Geometry: final body of the model. Coordinates: model frame, mm. Round coordinates to 2 decimals unless told otherwise and drop trailing zeros. Loops run counter-clockwise (first coordinate to the right, second up) from the corner with the lowest first, then second, coordinate; pieces in that order, holes last. Notation, with made-up numbers: (20, 76) - (68, 76) arc R23 ccw to (68, 93) - close; hole circle Ø5 at (-8, 76.5). An arc over 180 degrees is marked (long way). Write item = value, one per line. Start each with the question number.
Item 1: Section A-A (x = 5). Return loops of the section in (y, z).
Item 2: First-contact query: pin 1 (10 mm diameter, centred on y = 30.5, z = 30.5, fed in from +X); pin 2 (3 mm diameter, centred on y = 31.5, z = 99.5, fed in from +X); pin 3 (5 mm diameter, centred on x = 11, z = 122.5, fed in from -Y). Flat tips, straight axial feed; report the tip coordinate or a pass-through.
Item 3: Section C-C (z = 54). Return loops of the section in (x, y).
Item 4: Line query: line 1 (Z direction, x = 3.5, y = 28.5); line 2 (X direction, y = 20.5, z = 25); line 3 (Y direction, x = 1.75, z = 95.5) (3 decimals). Output: solid intervals per line, ascending. Write a range as from..to.
Item 5: Section B-B (y = 34.5). Return loops of the section in (x, z).
from build123d import *

# Parameters (mm, degrees)
F1_DEPTH = 12.7
F2_R     = 3.175
F3_DEPTH = 25.4
F5_DEPTH = 254


with BuildPart() as f1:
    # F0 (on Right) → F1 (new body)
    with BuildSketch(Plane.YZ):
        Polygon((19.05, 127), (0, 0), (38.1, 0), (38.1, 152.4), align=None)
    extrude(amount=F1_DEPTH)

    # F2 (on face) → F3 (cut)
    with BuildSketch(Plane(origin=(0, 0, 0), x_dir=(1, 0, 0), z_dir=(0, 0, -1))):
        with Locations((5.715, -22.225)):
            Circle(F2_R)
    extrude(amount=-F3_DEPTH, mode=Mode.SUBTRACT)

    # F4 (on face) → F5 (cut)
    with BuildSketch(Plane(origin=(0, 0, 0), x_dir=(1, 0, 0), z_dir=(0, 0, -1))):
        Polygon((6.35, 0), (12.7, -38.1), (12.7, 0), align=None)
    extrude(amount=-F5_DEPTH, mode=Mode.SUBTRACT)


solid = f1.part
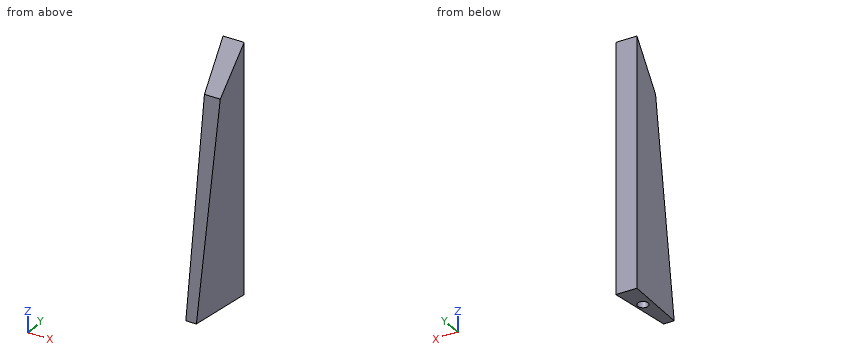
Taken from the geometry:
q1.outline = (0, 0) - (19.13, 0) - (19.13, 25.4) - (25.32, 25.4) - (25.32, 0) - (38.1, 0) - (38.1, 152.4) - (19.05, 127) - close
q2.pin_1 = 12.27
q2.pin_2 = 11.85
q2.pin_3 = 18.09
q3.outline = (0, 8.1) - (7.7, 8.1) - (12.7, 38.1) - (0, 38.1) - close
q4.line_1 = 0..139.6
q4.line_2 = 0..3.05, 8.38..9.77
q4.line_3 = 14.325..38.1
q5.outline = (0, 0) - (12.1, 0) - (12.1, 147.6) - (0, 147.6) - close
